from build123d import *

# Parameters (mm, degrees)
POCKET_DEPTH = 12


with BuildPart() as part:
    # Sketch → Revolution (revolve)
    with BuildSketch(Plane.XY):
        with BuildLine():
            Line((15, 31), (0, 31))
            Line((0, 31), (0, 0))
            Line((0, 0), (8, 0))
            Line((8, 0), (8, 6))
            Line((8, 6), (28, 6))
            Line((28, 18.5), (28, 6))
            ThreePointArc((28, 18.5), (24.163863, 27.520417), (15, 31))
        make_face()
    revolve(axis=Axis((0, 0, 0), (0, 1, 0)))

    # Sketch001 → Pocket (cut)
    with BuildSketch(Plane.XZ):
        with BuildLine():
            Line((-1.8, 2.523886), (1.8, 2.523886))
            ThreePointArc((-1.8, 2.523886), (0, -3.1), (1.8, 2.523886))
        make_face()
    extrude(amount=-POCKET_DEPTH, mode=Mode.SUBTRACT)


solid = part.part
Design review of the part built by this model. Coordinates are the model's own, in mm. A direction names the side the tool comes from. Give positions to 0.01 mm unless a question says otherwise; leave off trailing zeros. Order: outer loops, then holes, each group sorted by start corner. A loop starts at its lowest first (then second) coordinate and runs counter-clockwise, first axis right, second up. Notation, with made-up numbers: (-8.5, 79.25) - (8.5, 79.25) arc R15 cw to (8.5, 97.25) - close; hole circle Ø2 at (47, -32). An arc over 180 degrees is marked (long way). Use CSV: the item, a comma, the result in double quotes. Start each with the question number.
Q1. Take a section at D-D (y = 26.5). State the section outline as (x, z) points, and give its area (3 significant figures).
Q2. Take a section at C-C (y = 2.5). State the section outline as (x, z) points, and give its area (3 significant figures).
Q3. For P1, Ø10, axis at x = -1, z = -18.5, coming from the -Y side; P2, Ø8, axis at x = 5.5, z = -5.5, coming from the +Y side; P3, Ø1.8, axis at x = -0.5, y = 3.5, coming from the -Z side, all flat-tipped, find the tip position at first contact; note any pin that passes through.
Q4. For line 1 (Z direction, x = 0, y = 9.75); line 2 (Z direction, x = 0, y = 4); line 3 (X direction, y = 3, z = 0), list the stretches that pass through material, from the lowest coordinate up.
Q5. Take a section at B-B (z = 0). State the section outline as (x, y) points, and give its area (3 significant figures).
Q6. Machinability: for faces 1 (the face through (-1.73, 3.04, 7.81)), 2 (the face through (-3.4, 0, -0.1)), which of the approach directions +Z, -Z, +X, -X, +Y, -Y give a long, thin tool a straight path to every point of the face, cutting with its end or side? Answer none if there is none.
Q7. Draft analysis for pull direction Z (two halves, no side actions). For faces 3 (the face through (0, 12, 0)), 4 (the face through (25.865, 12.162, 10.724)), 5 (the face through (-6, 6, 6)), state which applies: pulls with the +Z half, pulls with the -Z half, needs draft (parallel to the pull), parting line crosses it, or undercut.
Q8. Take a section at A-A (x = 0). State the section outline as (y, z) points.
Calculated:
1,outline,"circle Ø50.23 at (0, 0)"
1,area,"1,980 mm²"
2,outline,"circle Ø16 at (0, 0); hole (-1.8, 2.52) arc R3.1 ccw (long way) to (1.8, 2.52) - close"
2,area,"172 mm²"
3,P1,"stops at y = 6"
3,P2,"stops at y = 31"
3,P3,"stops at z = -8"
4,line 1,"z = -28 to -3.1, 2.52 to 28"
4,line 2,"z = -8 to -3.1, 2.52 to 8"
4,line 3,"x = -8 to -3.1, 3.1 to 8"
5,outline,"(-28, 6) - (-8, 6) - (-8, 0) - (-3.1, 0) - (-3.1, 12) - (3.1, 12) - (3.1, 0) - (8, 0) - (8, 6) - (28, 6) - (28, 18.5) arc R12.5 ccw to (15, 31) - (-15, 31) arc R12.5 ccw to (-28, 18.5) - close"
5,area,"1,350 mm²"
6,face 1,"-Y"
6,face 2,"+Z, -Z, +X, -X, -Y"
7,face 3,"undercut"
7,face 4,"parting line crosses it"
7,face 5,"needs draft"
8,outline,"(0, -8) - (6, -8) - (6, -28) - (18.5, -28) arc R12.5 ccw to (31, -15) - (31, 15) arc R12.5 ccw to (18.5, 28) - (6, 28) - (6, 8) - (0, 8) - (0, 2.52) - (12, 2.52) - (12, -3.1) - (0, -3.1) - close"
